The drawing under review shows one solid part. Ordinate dimensions are in mm from its lowest x, y, z. A direction names the side the tool comes from. Give positions to 0.01 mm unless a question says otherwise; leave off trailing zeros. Write each loop counter-clockwise with the first axis right and the second up, starting at its lowest first coordinate (ties: lowest second). Pieces come first, ordered by that corner, then holes. Notation, with made-up numbers: (1, -24.5) -> (57, -24.5) arc R21 cw to (57, -8.5) -> close; hole circle Ø1 at (51, 16). An arc over 180 degrees is marked (long way). Use CSV: the item, a comma, the result in double quotes.
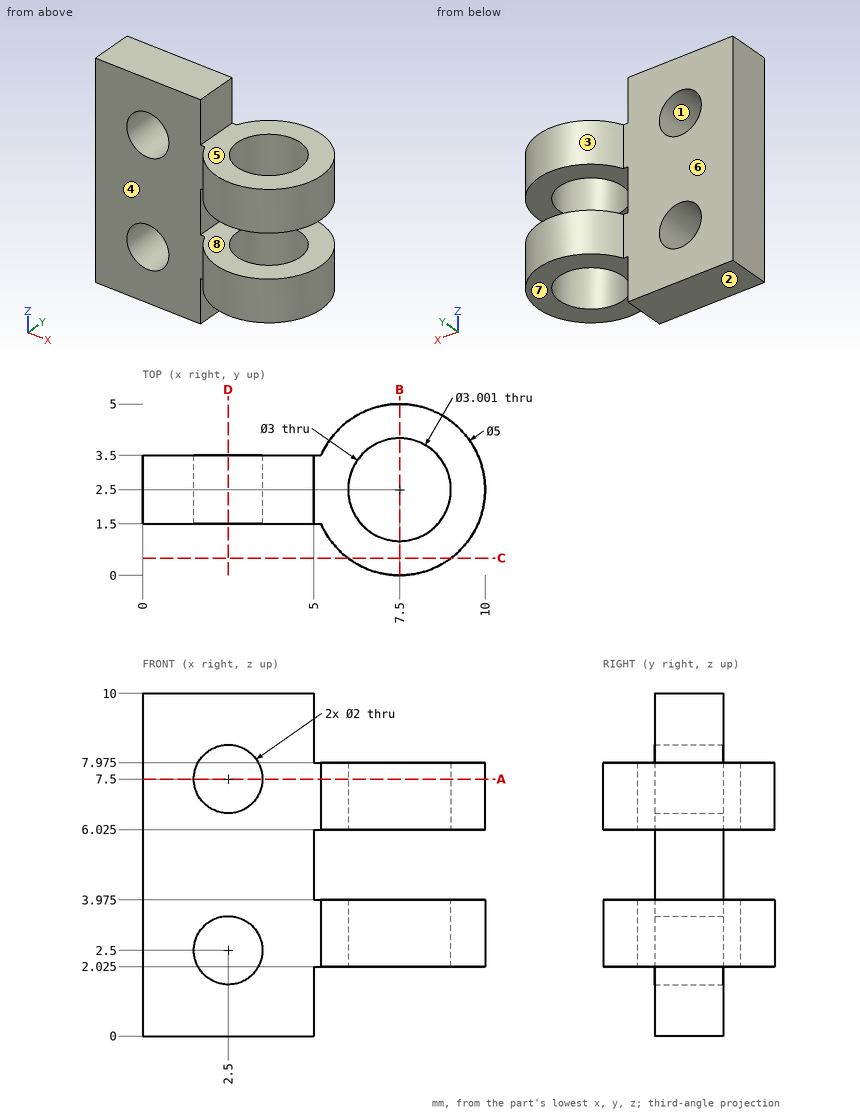
(1) Mouldability with a two-part tool opening along X and no side actions: class the marked faces 1, 2 and 3 as +X half, -X half, draft (parallel to the pull), parting line (faces both ways), or undercut.
Established:
face 1,"undercut"
face 2,"draft"
face 3,"parting line"
(2) Tool access review of the marked faces 4, 5, 6, 7 and 8: name each direction out of +Z, -Z, +X, -X, +Y, -Y from which nothing blocks a thin tool from reaching the whole face with its end or side.
Established:
face 4,"+Z, -Z, -X, -Y"
face 5,"+Z, +X, +Y, -Y"
face 6,"+Z, -Z, -X, +Y"
face 7,"-Z, +X, +Y, -Y"
face 8,"+X, +Y, -Y"
(3) For line 1 along X through (y, z) = (2.6, 2.5); line 2 along Z through (x, y) = (2.5, 2.3); line 3 along Z through (x, y) = (2, 2.6), list the stretches that pass through material, from the lowest coordinate up. Write a range as [from, to].
Established:
line 1,"x = [0, 1.5], [3.5, 6], [9, 10]"
line 2,"z = [0, 1.5], [3.5, 6.5], [8.5, 10]"
line 3,"z = [0, 1.63], [3.37, 6.63], [8.37, 10]"
(4) Take a section at B-B (x = 7.5). Write out the cut boundary in (y, z) (1 decimal).
Established:
outline,"(0, 2) -> (1, 2) -> (1, 4) -> (0, 4) -> close; (0, 6) -> (1, 6) -> (1, 8) -> (0, 8) -> close; (4, 2) -> (5, 2) -> (5, 4) -> (4, 4) -> close; (4, 6) -> (5, 6) -> (5, 8) -> (4, 8) -> close"
(5) Take a section at D-D (x = 2.5). Write out the cut boundary in (y, z).
Established:
outline,"(1.5, 0) -> (3.5, 0) -> (3.5, 1.5) -> (1.5, 1.5) -> close; (1.5, 3.5) -> (3.5, 3.5) -> (3.5, 6.5) -> (1.5, 6.5) -> close; (1.5, 8.5) -> (3.5, 8.5) -> (3.5, 10) -> (1.5, 10) -> close"
(6) Take a section at C-C (y = 0.5). Write out the cut boundary in (x, z) (3 decimals).
Established:
outline,"(6, 2.025) -> (9, 2.025) -> (9, 3.975) -> (6, 3.975) -> close; (6, 6.025) -> (9, 6.025) -> (9, 7.975) -> (6, 7.975) -> close"
(7) Take a section at A-A (z = 7.5). Write out the cut boundary in (x, y), then the cut area to 3 significant figures.
Established:
outline,"(0, 1.5) -> (1.5, 1.5) -> (1.5, 3.5) -> (0, 3.5) -> close; (3.5, 1.5) -> (5.21, 1.5) arc R2.5 ccw (long way) to (5.21, 3.5) -> (3.5, 3.5) -> close; hole circle Ø3 at (7.5, 2.5)"
area,"18.7 mm2"
(8) Clearance check with flat-ended pins moving along their axes: pin 1 (1.5 mm diameter, centred on x = 8, y = 4, fed in from -Z) (3 decimals); pin 2 (1.5 mm diameter, centred on x = 8.5, y = 3.5, fed in from +Z) (3 decimals); pin 3 (1.6 mm diameter, centred on x = 2, z = 7, fed in from +Y). State where each tip first meets the part, or that it passes through.
Established:
pin 1,"stops at z = 2.025"
pin 2,"stops at z = 7.975"
pin 3,"stops at y = 3.5"
